Read the model definition and answer for the solid it produces. Units are mm, in the model's axes. A direction names the side the tool comes from. Coordinates: 2 decimals unless noted, no trailing zeros. Loops run counter-clockwise (first coordinate to the right, second up) from the corner with the lowest first, then second, coordinate; pieces in that order, holes last.
from build123d import *

# Parameters (mm, degrees)
PLATE_DEPTH             = 4
SKETCH2_R               = 1.5
PLATE_MOUNTINGS_DEPTH   = 130.631207662
SKETCH3_R               = 1.5
LIGHT_SENSOR_DEPTH      = 130.631207662
SKETCH4_R               = 1.5
CUT_EXTRUDE3_DEPTH      = 130.631207662
MIRROR2_COPY_1_SKETCH_R = 1.5
MIRROR2_COPY_1_DEPTH    = 130.631207662


with BuildPart() as part:
    # Sketch1 → Plate (new body)
    with BuildSketch(Plane(origin=(0, 0, 0), x_dir=(1, 0, 0), z_dir=(0, 1, 0))):
        with BuildLine():
            Line((62, 4), (46.5, 4))
            Line((46.5, 4), (46.5, 75.5))
            Line((46.5, 75.5), (66, 75.5))
            ThreePointArc((66, 75.5), (0, 111.5), (-66, 75.5))
            Line((-66, 75.5), (-46.5, 75.5))
            Line((-46.5, 75.5), (-46.5, 4))
            Line((-46.5, 4), (-62, 4))
            ThreePointArc((-62, 4), (-66, 0), (-62, -4))
            Line((-62, -4), (-46.5, -4))
            Line((-46.5, -4), (-46.5, -75.5))
            Line((-46.5, -75.5), (-66, -75.5))
            ThreePointArc((-66, -75.5), (0, -111.5), (66, -75.5))
            Line((66, -75.5), (46.5, -75.5))
            Line((46.5, -75.5), (46.5, -4))
            Line((46.5, -4), (62, -4))
            ThreePointArc((62, -4), (66, 0), (62, 4))
        make_face()
    extrude(amount=PLATE_DEPTH)

    # Sketch2 → Plate mountings (cut, through all)
    with BuildSketch(Plane(origin=(0, 4, 0), x_dir=(1, 0, 0), z_dir=(0, 1, 0))):
        with Locations(Location((55, 0, 0), (0, 0, 270))):
            Circle(SKETCH2_R)
        with Locations(Location((55, 80, 0), (0, 0, 270))):
            Circle(SKETCH2_R)
        with Locations(Location((-55, 0, 0), (0, 0, 90))):
            Circle(SKETCH2_R)
        with Locations(Location((-55, 80, 0), (0, 0, 90))):
            Circle(SKETCH2_R)
        with Locations(Location((52.5, -84, 0), (0, 0, 270))):
            Circle(SKETCH2_R)
        with Locations(Location((-52.5, -84, 0), (0, 0, 90))):
            Circle(SKETCH2_R)
    extrude(amount=-PLATE_MOUNTINGS_DEPTH, mode=Mode.SUBTRACT)

    # Sketch3 → Light sensor (cut, through all)
    with BuildSketch(Plane(origin=(0, 4, 0), x_dir=(1, 0, 0), z_dir=(0, 1, 0))):
        with Locations(Location((-20, -89.5, 0), (0, 0, 270))):
            Circle(SKETCH3_R)
        with Locations(Location((0, -89.5, 0), (0, 0, 270))):
            Circle(SKETCH3_R)
        with Locations(Location((20, -89.5, 0), (0, 0, 270))):
            Circle(SKETCH3_R)
        with Locations(Location((0, -99.5, 0), (0, 0, 270))):
            Circle(SKETCH3_R)
        with Locations(Location((20, -99.5, 0), (0, 0, 270))):
            Circle(SKETCH3_R)
        with Locations(Location((-20, -99.5, 0), (0, 0, 270))):
            Circle(SKETCH3_R)
    extrude(amount=-LIGHT_SENSOR_DEPTH, mode=Mode.SUBTRACT)

    # Sketch4 → Cut-Extrude3 (cut, through all)
    with BuildSketch(Plane(origin=(0, 4, 0), x_dir=(1, 0, 0), z_dir=(0, 1, 0))):
        with Locations(Location((25.5, 64.35, 0), (0, 0, 270))):
            Circle(SKETCH4_R)
        with Locations(Location((25.5, 56.35, 0), (0, 0, 270))):
            Circle(SKETCH4_R)
    cut_extrude3 = extrude(amount=-CUT_EXTRUDE3_DEPTH, mode=Mode.SUBTRACT)

    # Mirror1: Cut-Extrude3 across plane
    add(cut_extrude3.mirror(Plane(origin=(0, 0, 0), x_dir=(0, 0, 1), z_dir=(1, 0, 0))), mode=Mode.SUBTRACT)

    # Mirror2: Cut-Extrude3 across plane
    add(cut_extrude3.mirror(Plane.XY), mode=Mode.SUBTRACT)

    # Mirror2 copy 1 sketch → Mirror2 copy 1 (cut, through all)
    with BuildSketch(Plane(origin=(0, 4, 0), x_dir=(-1, 0, 0), z_dir=(0, 1, 0))):
        with Locations(Location((25.5, 64.35, 0), (0, 0, 270))):
            Circle(MIRROR2_COPY_1_SKETCH_R)
        with Locations(Location((25.5, 56.35, 0), (0, 0, 270))):
            Circle(MIRROR2_COPY_1_SKETCH_R)
    extrude(amount=-MIRROR2_COPY_1_DEPTH, mode=Mode.SUBTRACT)


solid = part.part
Item 1: Find the intervals of material crossed by line 1 along X through (y, z) = (2.3, -80); line 2 along X through (y, z) = (2.9, 99.5); line 3 along X through (y, z) = (2.3, -64.35), in increasing order.
Numbers:
line 1: x = -62.87 to -56.5, -53.5 to 53.5, 56.5 to 62.87
line 2: x = -41.71 to -21.5, -18.5 to -1.5, 1.5 to 18.5, 21.5 to 41.71
line 3: x = -46.5 to -27, -24 to 24, 27 to 46.5
Item 2: A cutting plane is placed at A-A on y = 2.15. Give the number of separate pieces and of enclosed holes in the cut face, then the cut area to 3 significant figures.
Numbers:
separate pieces: 1
enclosed holes: 20
area: 20,900 mm2
Item 3: A cutting plane is placed at B-B on z = 12. Determine the outline of the cut face in (x, y), then the cut area to 3 significant figures.
Numbers:
outline: (-46.5, 0) - (46.5, 0) - (46.5, 4) - (-46.5, 4) - close
area: 372 mm2
Item 4: Which of the six approach directions +Z, -Z, +X, -X, +Y, -Y give full straight-line access (tool end or side, diameter ignored) to faces 1 (the face through (-56, 2, -75.5)), 2 (the face through (-1, 4, -2)), 3 (the face through (56, 2, -75.5))?
Numbers:
face 1: -X, +Y, -Y
face 2: +Z, -Z, +X, -X, +Y
face 3: +X, +Y, -Y
Item 5: A cutting plane is placed at C-C on x = 33. Determine the outline of the cut face in (y, z), then the cut area to 3 significant figures.
Numbers:
outline: (0, -104.23) - (4, -104.23) - (4, 104.23) - (0, 104.23) - close
area: 834 mm2
Item 6: Given pin 1 (2 mm diameter, centred on x = -55, y = 2, fed in from -Z); pin 2 (1.8 mm diameter, centred on x = -25.5, z = -64.35, fed in from -Y); pin 3 (2 mm diameter, centred on y = 2.5, z = 26, fed in from -X); pin 4 (1 mm diameter, centred on y = 0.5, z = -81.5, fed in from -X), each flat-ended and moving along its own axis, determine where each tip first touches the part or whether it passes through.
Numbers:
pin 1: stops at z = -89.98
pin 2: passes through
pin 3: stops at x = -46.5
pin 4: stops at x = -62.11
